Model file for the job. Use its own axes, mm. Face numbers are marked on the shaded views. Round coordinates to 2 decimals unless told otherwise and drop trailing zeros. Loops run counter-clockwise (first coordinate to the right, second up) from the corner with the lowest first, then second, coordinate; pieces in that order, holes last. Notation, with made-up numbers: (-25, 77) -> (-2, 77) arc R17 cw to (-2, 99) -> close; hole circle Ø10 at (29.25, 32). An arc over 180 degrees is marked (long way). Use a Markdown table: item, result.
from build123d import *

# Parameters (mm, degrees)
CROQUIS1_W              = 36.8
CROQUIS1_H              = 46.8
SALIENTE_EXTRUIR1_DEPTH = 1
CROQUIS2_W              = 8
CROQUIS2_H              = 2
SALIENTE_EXTRUIR2_DEPTH = 7
CROQUIS2_3_W            = 8
CROQUIS2_3_H            = 2
SALIENTE_EXTRUIR3_DEPTH = 7
CROQUIS6_R              = 1.5
CORTAR_EXTRUIR1_DEPTH   = 46.9


with BuildPart() as part:
    # Croquis1 → Saliente-Extruir1 (new body)
    with BuildSketch(Plane.XY):
        Rectangle(CROQUIS1_W, CROQUIS1_H)
    extrude(amount=SALIENTE_EXTRUIR1_DEPTH)

    # Croquis2 → Saliente-Extruir2 (add)
    with BuildSketch(Plane.XY):
        with Locations((0, 21.5)):
            Rectangle(CROQUIS2_W, CROQUIS2_H)
    extrude(amount=SALIENTE_EXTRUIR2_DEPTH)

    # Croquis2<3> → Saliente-Extruir3 (add)
    with BuildSketch(Plane.XY):
        with Locations((0, -21.5)):
            Rectangle(CROQUIS2_3_W, CROQUIS2_3_H)
    extrude(amount=SALIENTE_EXTRUIR3_DEPTH)

    # Croquis6 → Cortar-Extruir1 (cut, through all)
    with BuildSketch(Plane(origin=(0, 22.5, 0), x_dir=(1, 0, 0), z_dir=(0, 1, 0))):
        with Locations((0, -4)):
            Circle(CROQUIS6_R)
    extrude(amount=-CORTAR_EXTRUIR1_DEPTH, mode=Mode.SUBTRACT)


solid = part.part
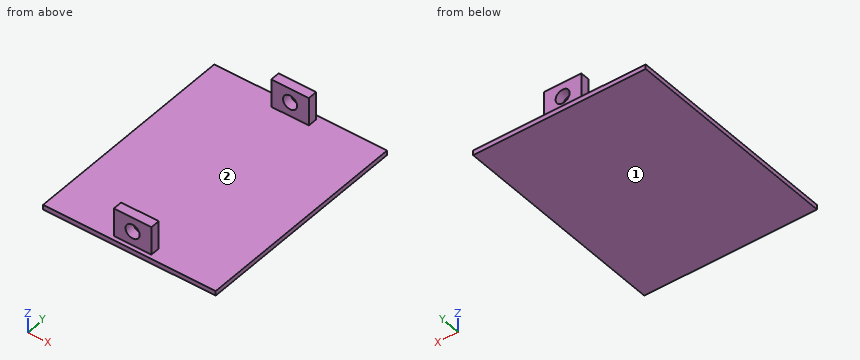
Q1. Band-saw the part on B-B, the plane x = 0. Give the cut face in (y, z), plus the area to 3 significant figures.
Results list:
| item | result |
|---|---|
| outline | (-23.4, 0) -> (23.4, 0) -> (23.4, 1) -> (22.5, 1) -> (22.5, 2.5) -> (20.5, 2.5) -> (20.5, 1) -> (-20.5, 1) -> (-20.5, 2.5) -> (-22.5, 2.5) -> (-22.5, 1) -> (-23.4, 1) -> close; (-22.5, 5.5) -> (-20.5, 5.5) -> (-20.5, 7) -> (-22.5, 7) -> close; (20.5, 5.5) -> (22.5, 5.5) -> (22.5, 7) -> (20.5, 7) -> close |
| area | 58.8 mm² |
Q2. Pull direction Y, two halves, no side cores. Call the marked faces 1 and 2: released by +Y, released by -Y, zero draft, split by the parting line, or undercut.
Results list:
| item | result |
|---|---|
| face 1 | zero draft |
| face 2 | undercut |
Q3. Band-saw the part on C-C, the plane y = 17. Give the cut face in (x, z), plus the area to 3 significant figures.
Results list:
| item | result |
|---|---|
| outline | (-18.4, 0) -> (18.4, 0) -> (18.4, 1) -> (-18.4, 1) -> close |
| area | 36.8 mm² |
Q4. Band-saw the part on A-A, the plane z = 4. Give the cut face in (x, y), plus the area to 3 significant figures.
Results list:
| item | result |
|---|---|
| outline | (-4, -22.5) -> (-1.5, -22.5) -> (-1.5, -20.5) -> (-4, -20.5) -> close; (-4, 20.5) -> (-1.5, 20.5) -> (-1.5, 22.5) -> (-4, 22.5) -> close; (1.5, -22.5) -> (4, -22.5) -> (4, -20.5) -> (1.5, -20.5) -> close; (1.5, 20.5) -> (4, 20.5) -> (4, 22.5) -> (1.5, 22.5) -> close |
| area | 20.0 mm² |
Q5. Drill centre lines: L1, parallel to Y at x = -2.5, z = 2.25; L2, parallel to Z at x = 0, y = 21.65; L3, parallel to X at y = 22.05, z = 4. Where is each one in solid material? Low to high. Write a range as from..to.
Results list:
| item | result |
|---|---|
| L1 | y = -22.5..-20.5, 20.5..22.5 |
| L2 | z = 0..2.5, 5.5..7 |
| L3 | x = -4..-1.5, 1.5..4 |
Q6. Band-saw the part on D-D, the plane x = -6. Give the cut face in (y, z).
Results list:
| item | result |
|---|---|
| outline | (-23.4, 0) -> (23.4, 0) -> (23.4, 1) -> (-23.4, 1) -> close |
Q7. Flat gauge pins, fed straight in: pin 1 (2 mm diameter, centred on y = 22, z = 2.5, fed in from +X); pin 2 (2 mm diameter, centred on x = 11, y = 9, fed in from +Z); pin 3 (3.5 mm diameter, centred on x = 0, z = 4, fed in from -Y). Where does each tip first touch, or does it go through?
Results list:
| item | result |
|---|---|
| pin 1 | stops at x = 4 |
| pin 2 | stops at z = 1 |
| pin 3 | stops at y = -22.5 |
